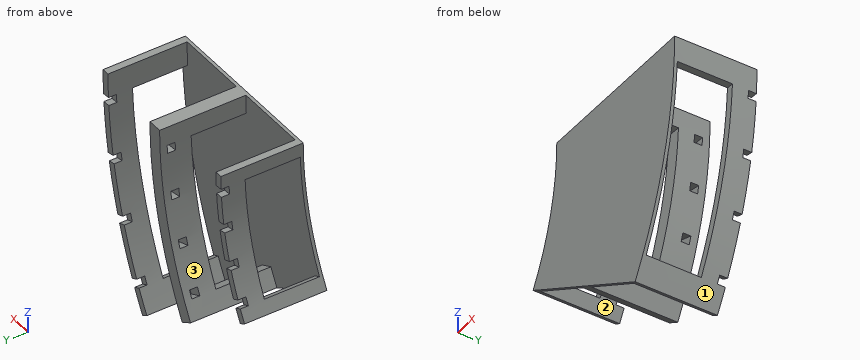
```python
from build123d import *

# Parameters (mm, degrees)
AUFSATZ_LINEAR_AUSTRAGEN1_DEPTH   = 51.5
AUFSATZ_LINEAR_AUSTRAGEN1_2_DEPTH = 51.5
AUFSATZ_LINEAR_AUSTRAGEN1_3_DEPTH = 51.5
SCHNITT_LINEAR_START              = -5
SCHNITT_LINEAR_AUSTRAGEN1_DEPTH   = 5
AUFSATZ_LINEAR_AUSTRAGEN2_DEPTH   = 2
SCHNITT_LINEAR_START_2            = -49.5
SCHNITT_LINEAR_AUSTRAGEN2_DEPTH   = 34.5
AUFSATZ_LINEAR_AUSTRAGEN3_DEPTH   = 4.5


with BuildPart() as part:
    # Skizze1 → Aufsatz-Linear austragen1 (new body)
    with BuildSketch(Plane(origin=(0, 0, 0), x_dir=(1, 0, 0), z_dir=(0, 1, 0))):
        with BuildLine():
            Line((165, 0), (169.6, 0))
            ThreePointArc((169.6, 0), (163.821020139, 43.895710049), (146.877908482, 84.8))
            Line((146.877908482, 84.8), (142.894191624, 82.5))
            ThreePointArc((142.894191624, 82.5), (159.377761338, 42.705142442), (165, 0))
        make_face()
    extrude(amount=AUFSATZ_LINEAR_AUSTRAGEN1_DEPTH)


with BuildPart() as body_2:
    # Skizze1 → Aufsatz-Linear austragen1 2 (new body)
    with BuildSketch(Plane(origin=(0, 0, 0), x_dir=(1, 0, 0), z_dir=(0, 1, 0))):
        with BuildLine():
            Line((215.5, 0), (224.5, 0))
            ThreePointArc((224.5, 0), (216.850348002, 58.104875626), (194.42270315, 112.25))
            Line((194.42270315, 112.25), (186.628474516, 107.75))
            ThreePointArc((186.628474516, 107.75), (208.157015565, 55.77550422), (215.5, 0))
        make_face()
    extrude(amount=AUFSATZ_LINEAR_AUSTRAGEN1_2_DEPTH)


with BuildPart() as body_3:
    # Skizze1 → Aufsatz-Linear austragen1 3 (new body)
    with BuildSketch(Plane(origin=(0, 0, 0), x_dir=(1, 0, 0), z_dir=(0, 1, 0))):
        with BuildLine():
            Line((234.173269183, 135.2), (238.156986041, 137.5))
            ThreePointArc((238.156986041, 137.5), (265.629602229, 71.175237403), (275, 0))
            Line((275, 0), (270.4, 0))
            ThreePointArc((270.4, 0), (261.186343429, 69.984669796), (234.173269183, 135.2))
        make_face()
    extrude(amount=AUFSATZ_LINEAR_AUSTRAGEN1_3_DEPTH)


with BuildPart() as schnitt_linear_austragen1_tool:
    # Skizze2 → Schnitt-Linear austragen1 (new body)
    with BuildSketch(Plane(origin=(0, 51.5, 0), x_dir=(1, 0, 0), z_dir=(0, 1, 0)).offset(SCHNITT_LINEAR_START)):
        with BuildLine():
            Line((164.464314583, 13.284924864), (274.236356527, 20.479764614))
            ThreePointArc((274.236356527, 20.479764614), (274.411203891, 17.985860538), (274.563372173, 15.490469997))
            Line((274.563372173, 15.490469997), (164.791330229, 8.295630248))
            ThreePointArc((164.791330229, 8.295630248), (164.646722334, 10.791516323), (164.464314583, 13.284924864))
        make_face()
        with BuildLine():
            Line((161.323268916, 34.638171229), (269.217080788, 56.099584774))
            ThreePointArc((269.217080788, 56.099584774), (269.715952111, 53.649838554), (270.192532398, 51.195658372))
            Line((270.192532398, 51.195658372), (162.298720527, 29.734244827))
            ThreePointArc((162.298720527, 29.734244827), (161.829571267, 32.189903133), (161.323268916, 34.638171229))
        make_face()
        with BuildLine():
            Line((157.029134718, 50.664098233), (261.198623482, 86.024874838))
            ThreePointArc((261.198623482, 86.024874838), (260.405785611, 88.395852958), (259.591426156, 90.759525485))
            Line((259.591426156, 90.759525485), (155.421937391, 55.398748881))
            ThreePointArc((155.421937391, 55.398748881), (156.243471367, 53.037511775), (157.029134718, 50.664098233))
        make_face()
        with BuildLine():
            Line((149.072736877, 70.727074872), (247.735533701, 119.382181845))
            ThreePointArc((247.735533701, 119.382181845), (246.640003921, 121.62938981), (245.52409025, 123.866545552))
            Line((245.52409025, 123.866545552), (146.861293426, 75.211438579))
            ThreePointArc((146.861293426, 75.211438579), (147.984002353, 72.977633886), (149.072736877, 70.727074872))
        make_face()
    extrude(amount=SCHNITT_LINEAR_AUSTRAGEN1_DEPTH)


with BuildPart() as part_1:
    add(part.part)

    # Schnitt-Linear austragen1: cut by schnitt_linear_austragen1_tool
    add(schnitt_linear_austragen1_tool.part, mode=Mode.SUBTRACT)



with BuildPart() as body_2_1:
    add(body_2.part)

    # Schnitt-Linear austragen1: cut by schnitt_linear_austragen1_tool
    add(schnitt_linear_austragen1_tool.part, mode=Mode.SUBTRACT)


with BuildPart() as body_3_1:
    add(body_3.part)

    # Schnitt-Linear austragen1: cut by schnitt_linear_austragen1_tool
    add(schnitt_linear_austragen1_tool.part, mode=Mode.SUBTRACT)


with BuildPart() as part_2:
    add(part_1.part)

    add(body_2_1.part)  # Aufsatz-Linear austragen2 merges body 2

    add(body_3_1.part)  # Aufsatz-Linear austragen2 merges body 3
    # Skizze4 → Aufsatz-Linear austragen2 (add)
    with BuildSketch(Plane.XZ):
        with BuildLine():
            Line((165, 0), (275, 0))
            ThreePointArc((275, 0), (265.629602229, -71.175237403), (238.156986041, -137.5))
            Line((238.156986041, -137.5), (142.894191624, -82.5))
            ThreePointArc((142.894191624, -82.5), (159.377761338, -42.705142442), (165, 0))
        make_face()
    extrude(amount=-AUFSATZ_LINEAR_AUSTRAGEN2_DEPTH)

    # Skizze5 → Schnitt-Linear austragen2 (cut)
    with BuildSketch(Plane(origin=(0, 51.5, 0), x_dir=(1, 0, 0), z_dir=(0, 1, 0)).offset(SCHNITT_LINEAR_START_2)):
        with BuildLine():
            Line((164.791330229, 8.295630248), (274.563372173, 15.490469997))
            ThreePointArc((274.563372173, 15.490469997), (265.629602229, 71.175237403), (245.52409025, 123.866545552))
            Line((245.52409025, 123.866545552), (146.861293426, 75.211438579))
            ThreePointArc((146.861293426, 75.211438579), (159.377761338, 42.705142442), (164.791330229, 8.295630248))
        make_face()
    extrude(amount=SCHNITT_LINEAR_AUSTRAGEN2_DEPTH, mode=Mode.SUBTRACT)

    # Skizze6 → Aufsatz-Linear austragen3 (add)
    with BuildSketch(Plane(origin=(0, 51.5, 0), x_dir=(1, 0, 0), z_dir=(0, 1, 0))):
        with BuildLine():
            Line((186.628474516, 107.75), (194.42270315, 112.25))
            ThreePointArc((194.42270315, 112.25), (216.850348002, 58.104875626), (224.5, 0))
            Line((224.5, 0), (215.5, 0))
            ThreePointArc((215.5, 0), (208.157015565, 55.77550422), (186.628474516, 107.75))
        make_face()
    extrude(amount=AUFSATZ_LINEAR_AUSTRAGEN3_DEPTH)


solid = part_2.part
```
Source: CAD feature listing. Evaluate the final solid. Frame: model axes, mm. Face numbers are marked on the shaded views. A direction names the side the tool comes from. Coordinates: 2 decimals unless noted, no trailing zeros. Loops run counter-clockwise (first coordinate to the right, second up) from the corner with the lowest first, then second, coordinate; pieces in that order, holes last. Notation, with made-up numbers: M 5,-5.5 L 46,-5.5 A10 ccw 46,-0.5 Z; hole C 1,12 d7. An arc over 180 degrees is marked long. Use a Markdown table: item, result. Add a question column.
Q1. Section query C-C, the plane y = 41. Return loops of the section in (x, z), and give its area (3 significant figures).
Q2. Section query B-B, the plane z = -115. Return loops of the section in (x, y), and give its area (3 significant figures).
Q3. Section query D-D, the plane x = 189.5. Return loops of the section in (y, z).
Q4. Access query for the marked faces 1, 2 and 3. Directions: +Z, -Z, +X, -X, +Y, -Y. A direction counts if a zero-diameter tool reaches every point of the face in a straight line with its end or side. Return the directions, or none.
Q5. First-contact query: pin 1 (6 mm diameter, centred on y = 40.5, z = -52, fed in from +X); pin 2 (1.6 mm diameter, centred on x = 163, z = -33.5, fed in from +Y); pin 3 (5.5 mm diameter, centred on x = 157, z = -64.5, fed in from +Y); pin 4 (5 mm diameter, centred on x = 221.5, z = -109, fed in from -Y). Flat tips, straight axial feed; report the tip coordinate or a pass-through.
Q6. Section query A-A, the plane y = 21. Return loops of the section in (x, z).
Q7. Material intervals for L1, parallel to Y at x = 199, z = -98.5; L2, parallel to X at y = 49.5, z = -66 (3 decimals); L3, parallel to Y at x = 257.5, z = -91, sorted ascending.
Result:
| question | item | result |
|---|---|---|
| 1 | outline | M 142.89,-82.5 L 146.88,-84.8 A169.6 ccw 169.6,0 L 165,0 A165 cw Z; M 186.63,-107.75 L 194.42,-112.25 A224.5 ccw 224.5,0 L 215.5,0 A215.5 cw Z; M 234.17,-135.2 L 238.16,-137.5 A275 ccw 275,0 L 270.4,0 A270.4 cw Z |
| 1 | area | 2,100 mm2 |
| 2 | outline | M 199.19,0 L 249.8,0 L 249.8,2 L 199.19,2 Z; M 244.73,36.5 L 249.8,36.5 L 249.8,51.5 L 244.73,51.5 Z |
| 2 | area | 177 mm2 |
| 3 | outline | M 0,-109.41 L 56,-109.41 L 56,-102.62 L 2,-102.62 L 2,0 L 0,0 Z |
| 4 | face 1 | -Z, +X, +Y, -Y |
| 4 | face 2 | -Z, +Y |
| 4 | face 3 | +Z, +Y |
| 5 | pin 1 | stops at x = 270.6 |
| 5 | pin 2 | stops at y = 46.5 |
| 5 | pin 3 | stops at y = 51.5 |
| 5 | pin 4 | stops at y = 0 |
| 6 | outline | M 142.89,-82.5 L 146.88,-84.8 A169.6 ccw 150.99,-77.25 L 146.86,-75.21 A165 cw Z; M 164.79,-8.3 L 169.38,-8.6 A169.6 ccw 169.6,0 L 165,0 A165 cw Z; M 186.63,-107.75 L 194.42,-112.25 A224.5 ccw 200.23,-101.53 L 192.16,-97.55 A215.5 cw Z; M 215.19,-11.6 L 224.17,-12.19 A224.5 ccw 224.5,0 L 215.5,0 A215.5 cw Z; M 234.17,-135.2 L 238.16,-137.5 A275 ccw 245.52,-123.87 L 241.4,-121.83 A270.4 cw Z; M 269.97,-15.19 L 274.56,-15.49 A275 ccw 275,0 L 270.4,0 A270.4 cw Z |
| 7 | L1 | y = 0 to 2, 36.5 to 46.5, 51.5 to 56 |
| 7 | L2 | x = 151.225 to 156.231, 205.144 to 214.579, 262.222 to 266.963 |
| 7 | L3 | y = 0 to 2, 36.5 to 51.5 |
